Verification items for the finished model (mm, model axes). A direction names the side the tool comes from. Coordinates: 2 decimals unless noted, no trailing zeros. Order: outer loops, then holes, each group sorted by start corner. A loop starts at its lowest first (then second) coordinate and runs counter-clockwise, first axis right, second up. Notation, with made-up numbers: (-20, -35) -> (31, -35) arc R23 ccw to (31, -27) -> close; hole circle Ø1 at (18.25, -21.5). An arc over 180 degrees is marked (long way). Write item = value, one per line. Start each with the question number.
from build123d import *

# Parameters (mm, degrees)
CUT_EXTRUDE_1_DEPTH = 2.5
FILLET_1_R          = 0.3
CHAMFER_1_SIZE      = 1


with BuildPart() as part:
    # Эскиз1 → Повернуть1 (revolve)
    with BuildSketch(Plane.XY):
        Polygon((0, 0), (0, 4.25), (5, 4.25), (5, 2.5), (30, 2.5), (30, 0), align=None)
    revolve(axis=Axis((30, 0, 0), (-1, 0, 0)))

    # Эскиз2 → Вырез-Вытянуть1 (cut)
    with BuildSketch(Plane.ZY):
        Polygon((-1.154700538, 2), (-2.309401077, 0), (-1.154700538, -2), (1.154700538, -2), (2.309401077, 0), (1.154700538, 2), align=None)
    extrude(amount=-CUT_EXTRUDE_1_DEPTH, mode=Mode.SUBTRACT)

    # Скругление1
    fillet_1_edges = [part.edges().sort_by_distance(p)[0] for p in [
        (5, -2.5, 0),
        (0, -4.25, 0),
    ]]
    fillet(fillet_1_edges, radius=FILLET_1_R)

    # Фаска1
    chamfer_1_edges = [part.edges().sort_by_distance(p)[0] for p in [
        (30, -2.5, 0),
    ]]
    chamfer(chamfer_1_edges, length=CHAMFER_1_SIZE)


solid = part.part
Item 1: Section check B-B (x = 19.75). Record the boundary of the cut face in (y, z).
Item 2: Mould release check, pull along Y, two halves, no side actions. Record for faces 4 (the flat face through (30, 0, 0)), 5 (the flat face through (1.23, 0.99, 1.74)), 6 (the cylindrical face through (17.32, -0.54, 2.44)): pulls with the +Y half, pulls with the -Y half, needs draft (parallel to the pull), parting line crosses it, or undercut.
Item 3: Section check A-A (z = 0). Record the boundary of the cut face in (x, y).
Item 4: Tool access check on faces 1 (the flat face through (5, 1, 3)), 2 (the cylindrical face through (2.683, 2.285, -3.584)), 3 (the flat face through (1, -2, 0)). Record the directions out of +Z, -Z, +X, -X, +Y, -Y that give a thin tool (end or side, any length) a straight path to the whole face; none if there is none.
Item 5: Thickness scan on line 1 (Y direction, x = 22.75, z = 1.5); line 2 (X direction, y = -2.25, z = -3); line 3 (X direction, y = 1.25, z = 0). Record the ranges inside material, lowest first.
Item 6: Gauge pin test, flat ends, axial feed: P1, Ø1, axis at x = 26.5, y = -2, coming from the +Z side; P2, Ø1, axis at x = 19, z = -2.5, coming from the -Y side; P3, Ø1.5, axis at x = 20, z = -1, coming from the +Y side. Record the tip position at first contact, or that the pin passes through.
Filled sheet:
q1.outline = circle Ø5 at (0, 0)
q2.face_4 = needs draft
q2.face_5 = undercut
q2.face_6 = parting line crosses it
q3.outline = (0, -3.95) arc R0.3 ccw to (0.3, -4.25) -> (5, -4.25) -> (5, -2.8) arc R0.3 cw to (5.3, -2.5) -> (29, -2.5) -> (30, -1.5) -> (30, 1.5) -> (29, 2.5) -> (5.3, 2.5) arc R0.3 cw to (5, 2.8) -> (5, 4.25) -> (0.3, 4.25) arc R0.3 ccw to (0, 3.95) -> (0, 2) -> (2.5, 2) -> (2.5, -2) -> (0, -2) -> close
q4.face_1 = +X
q4.face_2 = +X, -X
q4.face_3 = -X
q5.line_1 = -2 to 2
q5.line_2 = 0 to 5
q5.line_3 = 2.5 to 30
q6.P1 = 2
q6.P2 = -1.5
q6.P3 = 2.49
